Verification items for the finished model (mm, model axes). Face numbers are marked on the shaded views. Coordinates: 2 decimals unless noted, no trailing zeros. Loops run counter-clockwise (first coordinate to the right, second up) from the corner with the lowest first, then second, coordinate; pieces in that order, holes last. Notation, with made-up numbers: (82, 84.5) - (128, 84.5) arc R27 cw to (128, 112.5) - close; hole circle Ø5 at (73.5, 8). An arc over 180 degrees is marked (long way). Answer as CSV lines item,"result". Start each with the question number.
1. Release check for a two-part mould opening along Y. For the marked faces 1, 2 and 3 record: pulls with the +Y half, pulls with the -Y half, needs draft (parallel to the pull), parting line crosses it, or undercut.
2. Cross-section at A-A (y = 0). Enter the section's corners in (x, z) (3 decimals).
3. Material ranges on line 1 (Z direction, x = 4.3, y = 0); line 2 (Y direction, x = 4, z = 3.5); line 3 (Z direction, x = 0.5, y = 3.5), recorded low to high. Write a range as [from, to].
4. Gauge pin test, flat ends, axial feed: P1, Ø2, axis at x = 2, z = -6.5, coming from the +Y side; P2, Ø1.5, axis at x = 5, z = -2, coming from the -Y side; P3, Ø8, axis at y = 3, z = 0, coming from the -X side; P4, Ø3, axis at x = 5, z = 6, coming from the +Y side. Record the tip position at first contact, or that the pin passes through.
5. Cross-section at C-C (x = 3.4). Enter the section's corners in (y, z), plus the area to 3 significant figures.
6. Cross-section at B-B (x = 5.15). Enter the section's corners in (y, z), plus the area to 3 significant figures.
Autodesk Inventor part; units mm, degrees
ref_plane "Work Plane1" through (-22.2768, 0, 0) normal (0, -0.8660254, -0.5) x (1, 0, 0)
ref_plane "YZ Plane" through (0, 0, 0) normal (1, 0, 0) x (0, 1, 0)
ref_plane "XZ Plane" through (0, 0, 0) normal (0, 1, 0) x (-1, 0, 0)
sketch "Эскиз1" plane through (0, 0, 0) normal (1, 0, 0) x (0, 1, 0)
  line L0 (-10.3923, 0) -> (-5.1962, 9)
  line L1 (-5.1962, 9) -> (5.1962, 9)
  line L2 (5.1962, 9) -> (10.3923, 0)
  line L3 (10.3923, 0) -> (5.1962, -9)
  line L4 (5.1962, -9) -> (-5.1962, -9)
  line L5 (-5.1962, -9) -> (-10.3923, 0)
  point P0 (0, 0)
  point P1 (0, 0)
  dimension "d0" = 20.7846
extrude "Базовый элемент" add sketch "Эскиз1" along normal blind 6
sketch "Эскиз2" plane through (0, 0, 0) normal (0, 0, 1) x (1, 0, 0)
  line L0 (0, 5.1962) -> (0, 10.3923)
  line L1 (0, 10.3923) -> (6, 10.3923)
  line L2 (6, 5.1962) -> (6, 10.3923)
  line L3 (-1.2, 0) -> (7.2, 0)
  line L4 (1.1993, 10.3923) -> (0, 8.315)
  line L5 (4.8007, 10.3923) -> (6, 8.315)
  dimension "d3" = 30
  dimension "d4" = 30
  dimension "d5" = 16.63
  dimension "d6" = 16.63
revolve "Фаска1" cut sketch "Эскиз2" angle 360 about axis through (-10, 0, 0) along (1, 0, 0)
sketch "Эскиз3" plane through (6, 0, 0) normal (1, 0, 0) x (0, 0, -1)
  arc A0 (-0.625, -1.0825) -> (0.625, -1.0825) centre (0, 0) ccw
hole "Резьба" at (6, 0, 0) direction (-1, 0, 0) diameter 10.376 end through all
chamfer "Фаска2" distance 0.8119 angle 30 1 edges at (6, 0, 5.188) measured on face at (6, 7.1795, -0.8718)
chamfer "Фаска3" distance 0.8119 angle 30 1 edges at (0, 0, 5.188) measured on face at (0, 7.1795, -0.8718)
ref_plane "Work Plane1" through (-22.2768, 0, 0) normal (0, -0.8660254, -0.5) x (1, 0, 0)
equation "\"d0\" = 1.1547 * SW"
equation "\"d1\" = KOH"
equation "\"d3\" = ANG1"
equation "\"d4\" = ANG2"
equation "\"d5\" = SW0"
equation "\"d6\" = SW01"
equation "\"d8\" = -0.5 * GD1 + 0.5 * NND"
equation "\"d40\" = -0.5 * GD1 + 0.5 * NND"
equation "\"d10\" = -0.5 * GD1 + 0.5 * NND"
equation "\"d41\" = -0.5 * GD1 + 0.5 * NND"
equation "\"ANG1\" = 30deg"
equation "\"ANG2\" = 30deg"
equation "\"NND\" = 12"
equation "\"KOH\" = 6"
equation "\"SW\" = 18"
equation "\"SW0\" = 16.63"
equation "\"SW01\" = SW0"
equation "\"GUL\" = 0.541266 * PTC"
equation "\"LADI\" = 12.345"
equation "\"TOA\" = 30deg"
equation "\"FAWI\" = 30deg"
equation "\"PTC\" = 1.5"
equation "\"THREADDIA\" = 12"
equation "\"E0\" = 1.155 * SW"
equation "\"GAL\" = 0.541266 * PTC"
properties part number "Копия гайки M12x1.5-6H ГОСТ 5916-70" material "Сталь, мягкая"
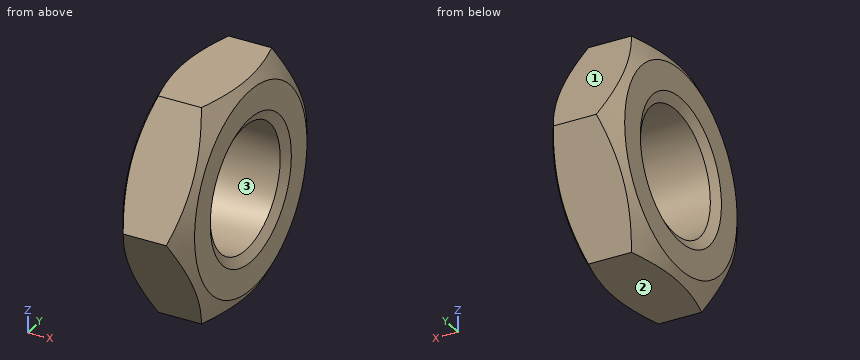
Values follow:
1,face 1,"pulls with the +Y half"
1,face 2,"needs draft"
1,face 3,"undercut"
2,outline,"(0, -8.315) - (0.395, -9) - (5.605, -9) - (6, -8.315) - (6, -6) - (5.531, -5.188) - (0.469, -5.188) - (0, -6) - close; (0, 6) - (0.469, 5.188) - (5.531, 5.188) - (6, 6) - (6, 8.315) - (5.605, 9) - (0.395, 9) - (0, 8.315) - close"
3,line 1,"z = [-9, -5.19], [5.19, 9]"
3,line 2,"y = [-8.37, -3.83], [3.83, 8.37]"
3,line 3,"z = [-8.49, -3.83], [3.83, 8.49]"
4,P1,"stops at y = 7.22"
4,P2,"stops at y = -9.67"
4,P3,"stops at x = 0"
4,P4,"stops at y = 7.79"
5,outline,"(-10.39, 0) - (-5.2, -9) - (5.2, -9) - (10.39, 0) - (5.2, 9) - (-5.2, 9) - close; hole circle Ø10.38 at (0, 0)"
5,area,"196 mm²"
6,outline,"(-9.72, -1.17) - (-5.87, -7.83) arc R9.79 ccw to (-3.85, -9) - (3.85, -9) arc R9.79 ccw to (5.87, -7.83) - (9.72, -1.17) arc R9.79 ccw to (9.72, 1.17) - (5.87, 7.83) arc R9.79 ccw to (3.85, 9) - (-3.85, 9) arc R9.79 ccw to (-5.87, 7.83) - (-9.72, 1.17) arc R9.79 ccw to start; hole circle Ø10.38 at (0, 0)"
6,area,"192 mm²"
